from build123d import *

# Parameters (mm, degrees)
F1_DEPTH = 3.175
F2_R     = 6.35
F5_D     = 13.49248


with BuildPart() as f1:
    # F0 (on Top) → F1 (new body, symmetric)
    with BuildSketch(Plane.XY):
        Polygon((-355.6, 50.8), (-355.6, -50.8), (-50.8, -50.8), (-50.8, -355.6), (50.8, -355.6), (355.6, -50.8), (355.6, 50.8), (50.8, 355.6), (-50.8, 355.6), align=None)
    extrude(amount=F1_DEPTH, both=True)

    # F2
    f2_edges = [f1.edges().sort_by_distance(p)[0] for p in [
        (-50.8, -50.8, 0),
    ]]
    fillet(f2_edges, radius=F2_R)

    # F5 (through all)
    with Locations(Plane.XY.offset(3.175)):
        with Locations((0, -254), (0, -152.4), (152.4, 0), (254, 0), (0, 152.4), (0, 254), (-152.4, 0), (-254, 0)):
            Hole(F5_D / 2)


solid = f1.part
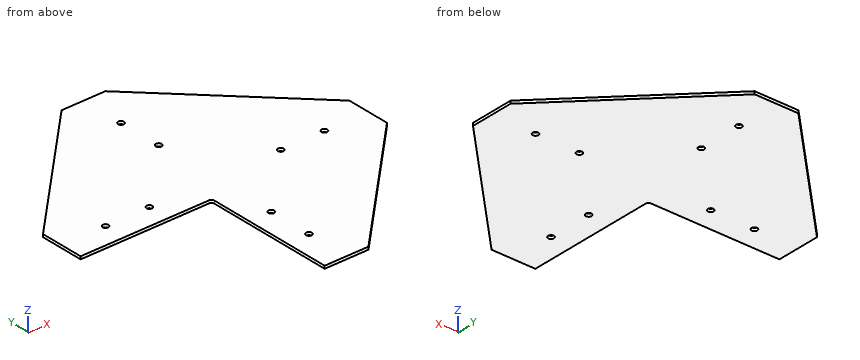
Input: part model. Units: mm. Frame: model coordinates. Round coordinates to 2 decimals unless told otherwise and drop trailing zeros. Write each loop counter-clockwise with the first axis right and the second up, starting at its lowest first coordinate (ties: lowest second). Pieces come first, ordered by that corner, then holes.
1) Ray query, L1, parallel to Y at x = 0, z = 0.75; L2, parallel to Y at x = -254, z = 1; L3, parallel to Y at x = -152.4, z = 0.5. Return the intervals inside material, ascending.
2) Cut plane B-B (x = -182.5). Return the cut outline in (y, z) (3 decimals).
3) Contact query for flat-ended pins moving along their axis: P1, Ø17.5, axis at x = 254, y = 0, coming from the +Z side (3 decimals); P2, Ø12, axis at x = 0, y = 254, coming from the -Z side; P3, Ø3, axis at x = -247.5, z = -1, coming from the -Y side; P4, Ø2, axis at y = -139.5, z = 2, coming from the -X side. Output: stop coordinate, or through.
4) Cut plane A-A (y = 76). Return the cut outline in (x, z) (3 decimals), then the cut area to 3 significant figures.
Geometry says:
1. L1: y = -355.6 to -260.75, -247.25 to -159.15, -145.65 to 145.65, 159.15 to 247.25, 260.75 to 355.6
1. L2: y = -50.8 to -6.75, 6.75 to 152.4
1. L3: y = -50.8 to -6.75, 6.75 to 254
2. outline: (-50.8, -3.175) - (223.9, -3.175) - (223.9, 3.175) - (-50.8, 3.175) - close
3. P1: stops at z = 3.175
3. P2: passes through
3. P3: stops at y = -50.8
3. P4: stops at x = -50.8
4. outline: (-330.4, -3.175) - (330.4, -3.175) - (330.4, 3.175) - (-330.4, 3.175) - close
4. area: 4,200 mm2
